Verification items for the finished model (mm, model axes). Face numbers are marked on the shaded views. A direction names the side the tool comes from. Coordinates: 2 decimals unless noted, no trailing zeros. Write each loop counter-clockwise with the first axis right and the second up, starting at its lowest first coordinate (ties: lowest second). Pieces come first, ordered by that corner, then holes. Notation, with made-up numbers: (-5, 36.5) -> (38, 36.5) arc R23 ccw to (38, 71.5) -> close; hole circle Ø7 at (6.25, 87.25). An arc over 180 degrees is marked (long way). Use a Markdown table: item, result. Add a question column.
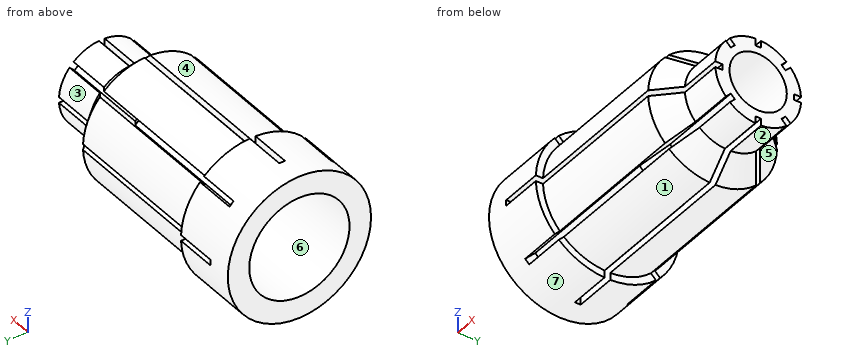
from build123d import *

# Parameters (mm, degrees)
CUT_EXTRUDE2_DEPTH = 0.2
CIRPATTERN2_COUNT  = 8
SKETCH4_W          = 0.4
SKETCH4_H          = 0.75
CUT_EXTRUDE3_DEPTH = 1
CIRPATTERN3_COUNT  = 8


with BuildPart() as part:
    # Sketch1 → Revolve1 (revolve)
    with BuildSketch(Plane.XY):
        Polygon((-10, 3), (-10, 2), (-16, 2), (-17.5, 3.5), (-29.5, 3.5), (-29.5, 5), (-24.88, 5), (-24.88, 4.5), (-14.5, 4.5), (-13, 3), align=None)
    revolve(axis=Axis((0, 0, 0), (-1, 0, 0)))

    # Sketch3 → Cut-Extrude2 (cut, symmetric)
    with BuildSketch(Plane.XY):
        Polygon((-14.5, 4.5), (-13, 3), (-10, 3), (-10, 2.5), (-16, 2.5), (-17.5, 4), (-27.8, 4), (-27.8, 5.5), (-24.88457259, 5.5), (-24.88457259, 4.5), align=None)
    cut_extrude2 = extrude(amount=CUT_EXTRUDE2_DEPTH, both=True, mode=Mode.SUBTRACT)

    # CirPattern2: Cut-Extrude2 ×8 about axis
    cirpattern2_axis = Axis((0, 0, 0), (1, 0, 0))
    for i in range(1, CIRPATTERN2_COUNT):
        add(cut_extrude2.rotate(cirpattern2_axis, i * 360 / CIRPATTERN2_COUNT), mode=Mode.SUBTRACT)

    # Sketch4 → Cut-Extrude3 (cut)
    with BuildSketch(Plane(origin=(-24.88, 0, 0), x_dir=(0, 0, -1), z_dir=(1, 0, 0))):
        with Locations((0, 4.872999199)):
            Rectangle(SKETCH4_W, SKETCH4_H)
    cut_extrude3 = extrude(amount=-CUT_EXTRUDE3_DEPTH, mode=Mode.SUBTRACT)

    # CirPattern3: Cut-Extrude3 ×8 about axis
    cirpattern3_axis = Axis((-24.88, 0, 0), (1, 0, 0))
    for i in range(1, CIRPATTERN3_COUNT):
        add(cut_extrude3.rotate(cirpattern3_axis, i * 360 / CIRPATTERN3_COUNT), mode=Mode.SUBTRACT)


solid = part.part
1) Set-up check for the marked faces 1, 2 and 3: record each of +Z, -Z, +X, -X, +Y, -Y from which the full face is reachable in a straight line by a thin tool's end or side.
2) Thickness scan on L1, parallel to Y at x = -13.1, z = 0; L2, parallel to Y at x = -23.25, z = 0. Record the ranges inside material, lowest first.
3) Release check for a two-part mould opening along Y. For the marked faces 4, 5, 6 and 7 record: released by +Y, released by -Y, zero draft, split by the parting line, or undercut.
4) Cross-section at A-A on z = 0. Record the boundary of the cut face in (x, y).
5) Gauge pin test, flat ends, axial feed: pin 1 (2 mm diameter, centred on x = -17.5, z = 3, fed in from +Y); pin 2 (6 mm diameter, centred on x = -14, y = 3.5, fed in from +Z); pin 3 (3 mm diameter, centred on x = -17.5, y = 0.5, fed in from -Z). Record the tip position at first contact, or that the pin passes through.
Returned:
| question | item | result |
|---|---|---|
| 1 | face 1 | -Z, +X, -Y |
| 1 | face 2 | -Z, +X, +Y |
| 1 | face 3 | +Z, +X, +Y |
| 2 | L1 | y = -2.5 to -2, 2 to 2.5 |
| 2 | L2 | y = -4 to -3.5, 3.5 to 4 |
| 3 | face 4 | released by -Y |
| 3 | face 5 | released by +Y |
| 3 | face 6 | undercut |
| 3 | face 7 | split by the parting line |
| 4 | outline | (-29.5, -5) -> (-27.8, -5) -> (-27.8, -4) -> (-17.5, -4) -> (-16, -2.5) -> (-10, -2.5) -> (-10, -2) -> (-16, -2) -> (-17.5, -3.5) -> (-29.5, -3.5) -> close; (-29.5, 3.5) -> (-17.5, 3.5) -> (-16, 2) -> (-10, 2) -> (-10, 2.5) -> (-16, 2.5) -> (-17.5, 4) -> (-27.8, 4) -> (-27.8, 5) -> (-29.5, 5) -> close |
| 5 | pin 1 | stops at y = 4.03 |
| 5 | pin 2 | stops at z = 4.47 |
| 5 | pin 3 | stops at z = -4.5 |
